from build123d import *

# Parameters (mm, degrees)
F1_DEPTH = 15
F2_R     = 32.5
F3_DEPTH = 15
F4_R     = 3.3
F5_DEPTH = 30


# Not quite as in the source:
# - a feature names something its author has since deleted; it is built from what else it names


with BuildPart() as f1:
    # F0 (on Top) → F1 (new body)
    with BuildSketch(Plane.XY):
        Polygon((0.369179663, 43.2996963774), (-37.3140472075, 21.9695671555), (-37.6832268705, -21.330129222), (-0.369179663, -43.2996963774), (37.3140472075, -21.9695671555), (37.6832268705, 21.330129222), align=None)
    extrude(amount=F1_DEPTH)

    # F2 (on face) → F3 (join)
    with BuildSketch(Plane.XY.offset(15)):
        Circle(F2_R)
    extrude(amount=F3_DEPTH)


with BuildPart() as f5:
    # F4 (on Top) → F5 (new body)
    with BuildSketch(Plane.XY):
        Circle(F4_R)
    extrude(amount=F5_DEPTH)


with BuildPart() as f1_1:
    add(f1.part)

    # F6: cut F5
    add(f5.part, mode=Mode.SUBTRACT)


solid = f1_1.part
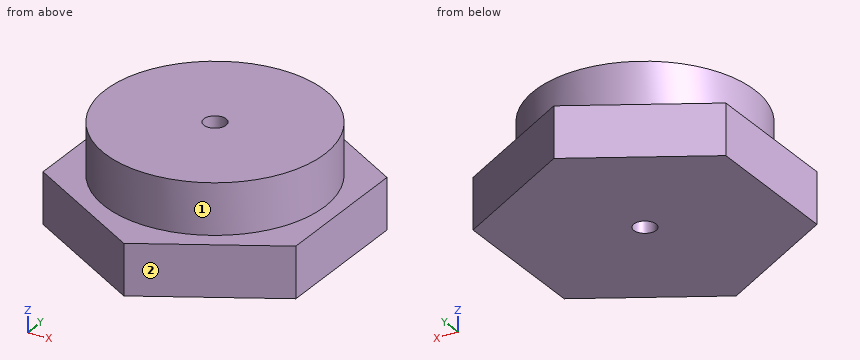
Model file for the job. Use its own axes, mm. Face numbers are marked on the shaded views. A direction names the side the tool comes from. Round coordinates to 2 decimals unless told otherwise and drop trailing zeros. Loops run counter-clockwise (first coordinate to the right, second up) from the corner with the lowest first, then second, coordinate; pieces in that order, holes last. Notation, with made-up numbers: M 40,-22.5 L 95,-22.5 A9 cw 95,-8.5 Z; hole C 63,80.25 d6. An arc over 180 degrees is marked long. One line per question, with ' | ' between items.
1) Flat gauge pins, fed straight in: pin 1 (1 mm diameter, centred on x = -6, y = -32.5, fed in from +Z); pin 2 (3 mm diameter, centred on y = -31.5, z = 9, fed in from -X); pin 3 (6 mm diameter, centred on y = -8, z = 4, fed in from +X). Where does each tip first touch, or does it go through?
Solved:
pin 1: stops at z = 15 | pin 2: stops at x = -22.96 | pin 3: stops at x = 37.46
2) Drill centre lines: line 1 along Y through (x, z) = (0, 20); line 2 along Y through (x, z) = (0, 11.75); line 3 along Y through (x, z) = (24.5, 21.5). Where is each one in solid material? Low to high.
Solved:
line 1: y = -32.5 to -3.3, 3.3 to 32.5 | line 2: y = -43.09 to -3.3, 3.3 to 43.09 | line 3: y = -21.35 to 21.35
3) Band-saw the part on A-A (z = 10). Give the cut face in (x, y).
Solved:
outline: M -37.68,-21.33 L -0.37,-43.3 L 37.31,-21.97 L 37.68,21.33 L 0.37,43.3 L -37.31,21.97 Z; hole C 0,0 d6.6
4) Band-saw the part on B-B (y = 0). Give the cut face in (x, z).
Solved:
outline: M -37.5,0 L -3.3,0 L -3.3,30 L -32.5,30 L -32.5,15 L -37.5,15 Z; M 3.3,0 L 37.5,0 L 37.5,15 L 32.5,15 L 32.5,30 L 3.3,30 Z
5) Band-saw the part on D-D (y = -36.5). Give the cut face in (x, z), then the cut area to 3 significant figures.
Solved:
outline: M -11.92,0 L 11.64,0 L 11.64,15 L -11.92,15 Z | area: 353 mm²
6) 3-axis set-ups, long thin cutter, end or side, ignore diameter. For the marked faces 1 and 2: which of +Z, -Z, +X, -X, +Y, -Y reach the whole face in a straight line?
Solved:
face 1: +Z | face 2: +Z, -Z, +X, -Y
7) Band-saw the part on C-C (x = -5.5). Give the cut face in (y, z), then the cut area to 3 significant figures.
Solved:
outline: M -40.28,0 L 39.98,0 L 39.98,15 L 32.03,15 L 32.03,30 L -32.03,30 L -32.03,15 L -40.28,15 Z | area: 2,160 mm²
